from build123d import *

# Parameters (mm, degrees)
SKETCH1_W           = 69.85
SKETCH1_H           = 12.7
BOSS_EXTRUDE1_DEPTH = 5.08
SKETCH2_W           = 9.525
SKETCH2_H           = 5.08
BOSS_EXTRUDE2_DEPTH = 5.08
SKETCH3_W           = 5.08
SKETCH3_H           = 6.35
CUT_EXTRUDE1_DEPTH  = 5.08


with BuildPart() as part:
    # Sketch1 → Boss-Extrude1 (new body)
    with BuildSketch(Plane.XY):
        Rectangle(SKETCH1_W, SKETCH1_H)
    extrude(amount=BOSS_EXTRUDE1_DEPTH)

    # Sketch2 → Boss-Extrude2 (add)
    with BuildSketch(Plane.XY.offset(5.08)):
        with Locations((-30.1625, 8.89)):
            Rectangle(SKETCH2_W, SKETCH2_H)
        with Locations((30.1625, 8.89)):
            Rectangle(SKETCH2_W, SKETCH2_H)
        with Locations((0, 8.89)):
            Rectangle(SKETCH2_W, SKETCH2_H)
    boss_extrude2 = extrude(amount=-BOSS_EXTRUDE2_DEPTH)

    # Mirror1: Boss-Extrude2 across plane
    add(boss_extrude2.mirror(Plane.ZX))

    # Sketch3 → Cut-Extrude1 (cut)
    with BuildSketch(Plane.XY.offset(5.08)):
        with Locations((-32.385, 0)):
            Rectangle(SKETCH3_W, SKETCH3_H)
        with Locations((32.385, 0)):
            Rectangle(SKETCH3_W, SKETCH3_H)
    extrude(amount=-CUT_EXTRUDE1_DEPTH, mode=Mode.SUBTRACT)


solid = part.part
The model under review builds one solid part; all positions refer to its coordinate system, in mm. A direction names the side the tool comes from. Give positions to 0.01 mm unless a question says otherwise; leave off trailing zeros. Order: outer loops, then holes, each group sorted by start corner. A loop starts at its lowest first (then second) coordinate and runs counter-clockwise, first axis right, second up. Notation, with made-up numbers: (40, 79.5) -> (90, 79.5) arc R18 cw to (90, 88.5) -> close; hole circle Ø7 at (-15.75, 69). An arc over 180 degrees is marked (long way). Write item = value, one per line. Start each with the question number.
(1) For L1, parallel to X at y = 6.75, z = 2.75 (1 decimal); L2, parallel to Y at x = -31, z = 0.4 (3 decimals); L3, parallel to Y at x = -11, z = 0.25, list the stretches that pass through material, from the lowest coordinate up. Write a range as from..to.
(2) For pin 1 Ø2 at (x, z) = (-19.5, 4.5) entering from +Y; pin 2 Ø1.5 at (y, z) = (0.5, 3.5) entering from -X (3 decimals), all flat-tipped, find the tip position at first contact; note any pin that passes through.
(3) Take a section at A-A (y = -7). Write out the cut boundary in (x, z) (1 decimal), plus the area to 3 significant figures.
(4) Take a section at D-D (y = -1.5). Write out the cut boundary in (x, z) (3 decimals), plus the area to 3 significant figures.
(5) Draft analysis for pull direction X (two halves, no side actions). For faces 1 (the flat face through (4.762, -9, 3)), 2 (the flat face through (34.925, 7, 3)), 3 (the flat face through (0, 11.43, 3)), state which applies: +X half, -X half, draft (parallel to the pull), parting line (faces both ways), or undercut.
(6) Tool access review of faces 4 (the flat face through (15, 6.35, 3)), 5 (the flat face through (25.4, -9, 3)), 6 (the flat face through (32, 3.175, 3)): name each direction out of +Z, -Z, +X, -X, +Y, -Y from which nothing blocks a thin tool from reaching the whole face with its end or side.
(7) Take a section at C-C (x = 20). Write out the cut boundary in (y, z), plus the area to 3 significant figures.
Returned:
q1.L1 = -34.9..-25.4, -4.8..4.8, 25.4..34.9
q1.L2 = -11.43..-3.175, 3.175..11.43
q1.L3 = -6.35..6.35
q2.pin_1 = 6.35
q2.pin_2 = -29.845
q3.outline = (-34.9, 0) -> (-25.4, 0) -> (-25.4, 5.1) -> (-34.9, 5.1) -> close; (-4.8, 0) -> (4.8, 0) -> (4.8, 5.1) -> (-4.8, 5.1) -> close; (25.4, 0) -> (34.9, 0) -> (34.9, 5.1) -> (25.4, 5.1) -> close
q3.area = 145 mm²
q4.outline = (-29.845, 0) -> (29.845, 0) -> (29.845, 5.08) -> (-29.845, 5.08) -> close
q4.area = 303 mm²
q5.face_1 = undercut
q5.face_2 = +X half
q5.face_3 = draft
q6.face_4 = +Z, -Z, +Y
q6.face_5 = +Z, -Z, -Y
q6.face_6 = +Z, -Z, +X
q7.outline = (-6.35, 0) -> (6.35, 0) -> (6.35, 5.08) -> (-6.35, 5.08) -> close
q7.area = 64.5 mm²
